Read the model definition and answer for the solid it produces. Units are mm, in the model's axes. Give positions to 0.01 mm unless a question says otherwise; leave off trailing zeros. Order: outer loops, then holes, each group sorted by start corner. A loop starts at its lowest first (then second) coordinate and runs counter-clockwise, first axis right, second up.
```python
from build123d import *

# Parameters (mm, degrees)
SKETCH1_W           = 25.4
SKETCH1_H           = 91.44
BOSS_EXTRUDE1_DEPTH = 3.175
SKETCH2_R           = 2.5527
SKETCH2_R_2         = 4.7625
CUT_EXTRUDE1_DEPTH  = 3.175
SKETCH3_R           = 1.651
SKETCH3_R_2         = 7.62
CUT_EXTRUDE2_DEPTH  = 3.175


with BuildPart() as part:
    # Sketch1 → Boss-Extrude1 (new body)
    with BuildSketch(Plane.XY):
        with Locations((12.7, 45.72)):
            Rectangle(SKETCH1_W, SKETCH1_H)
    extrude(amount=BOSS_EXTRUDE1_DEPTH)

    # Sketch2 → Cut-Extrude1 (cut)
    with BuildSketch(Plane.XY.offset(3.175)):
        with Locations((12.7, 6.35)):
            Circle(SKETCH2_R)
        with Locations((12.7, 38.1)):
            Circle(SKETCH2_R)
        with Locations((12.7, 22.225)):
            Circle(SKETCH2_R_2)
    extrude(amount=-CUT_EXTRUDE1_DEPTH, mode=Mode.SUBTRACT)

    # Sketch3 → Cut-Extrude2 (cut)
    with BuildSketch(Plane.XY.offset(3.175)):
        with Locations((12.7, 85.09)):
            Circle(SKETCH3_R)
        with Locations((12.7, 60.325)):
            Circle(SKETCH3_R)
        with Locations((12.7, 72.7075)):
            Circle(SKETCH3_R_2)
    extrude(amount=-CUT_EXTRUDE2_DEPTH, mode=Mode.SUBTRACT)


solid = part.part
```
1) For a pull along X with two mould halves and no side action, classify faces 1 (the face through (16.22, 65.95, 1.61)), 2 (the face through (0, 45, 2)), 3 (the face through (13, 0, 2)), 4 (the face through (25.4, 45, 2)) as released by +X, released by -X, zero draft, split by the parting line, or undercut.
Final values:
face 1: undercut
face 2: released by -X
face 3: zero draft
face 4: released by +X
2) The part is cut by section A-A on x = 12.7. Determine the outline of the cut face in (y, z) (1 decimal).
Final values:
outline: (0, 0) - (3.8, 0) - (3.8, 3.2) - (0, 3.2) - close; (8.9, 0) - (17.5, 0) - (17.5, 3.2) - (8.9, 3.2) - close; (27, 0) - (35.5, 0) - (35.5, 3.2) - (27, 3.2) - close; (40.7, 0) - (58.7, 0) - (58.7, 3.2) - (40.7, 3.2) - close; (62, 0) - (65.1, 0) - (65.1, 3.2) - (62, 3.2) - close; (80.3, 0) - (83.4, 0) - (83.4, 3.2) - (80.3, 3.2) - close; (86.7, 0) - (91.4, 0) - (91.4, 3.2) - (86.7, 3.2) - close
3) The part is cut by section D-D on z = 2.05. Count the separate pieces of the cut face and the enclosed holes in it, and give its area (3 significant figures).
Final values:
separate pieces: 1
enclosed holes: 6
area: 2,010 mm2
4) The part is cut by section C-C on x = 9. Determine the outline of the cut face in (y, z) (3 decimals).
Final values:
outline: (0, 0) - (19.226, 0) - (19.226, 3.175) - (0, 3.175) - close; (25.224, 0) - (66.046, 0) - (66.046, 3.175) - (25.224, 3.175) - close; (79.369, 0) - (91.44, 0) - (91.44, 3.175) - (79.369, 3.175) - close
5) Consider L1, parallel to Y at x = 14.75, z = 2.4; L2, parallel to X at y = 72.5, z = 2.5; L3, parallel to Y at x = 16.25, z = 1.15. Determine where each line is inside the solid, lowest interval first.
Final values:
L1: y = 0 to 4.83, 7.87 to 17.93, 26.52 to 36.58, 39.62 to 65.37, 80.05 to 91.44
L2: x = 0 to 5.08, 20.32 to 25.4
L3: y = 0 to 19.05, 25.4 to 65.96, 79.45 to 91.44
6) The part is cut by section B-B on y = 38.1. Determine the outline of the cut face in (x, z) (3 decimals).
Final values:
outline: (0, 0) - (10.147, 0) - (10.147, 3.175) - (0, 3.175) - close; (15.253, 0) - (25.4, 0) - (25.4, 3.175) - (15.253, 3.175) - close
